Could you check a few things on this model? Use its own coordinates, in mm. A direction names the side the tool comes from. Coordinates: 2 decimals unless noted, no trailing zeros. Write each loop counter-clockwise with the first axis right and the second up, starting at its lowest first coordinate (ties: lowest second). Pieces come first, ordered by that corner, then holes. Notation, with made-up numbers: M 72.25,38 L 130.25,38 A18 cw 130.25,53 Z; hole C 3,57 d7. An arc over 180 degrees is marked long. Write item = value, one per line.
```python
from build123d import *

# Parameters (mm, degrees)
SKETCH_1_R          = 72.5
SKETCH_1_R_2        = 50
EXTRUDE_1_DEPTH     = 13
SKETCH_2_R          = 65
SKETCH_2_R_2        = 55
CUT_EXTRUDE_1_DEPTH = 10


with BuildPart() as part:
    # 草图1 → 凸台-拉伸1 (new body)
    with BuildSketch(Plane(origin=(0, 0, 0), x_dir=(1, 0, 0), z_dir=(0, 1, 0))):
        with Locations(Location((0, 0, 0), (0, 0, 90))):
            Circle(SKETCH_1_R)
        with Locations(Location((0, 0, 0), (0, 0, 90))):
            Circle(SKETCH_1_R_2, mode=Mode.SUBTRACT)
    extrude(amount=EXTRUDE_1_DEPTH)

    # 草图2 → 切除-拉伸1 (cut)
    with BuildSketch(Plane(origin=(0, 13, 0), x_dir=(1, 0, 0), z_dir=(0, 1, 0))):
        with Locations(Location((0, 0, 0), (0, 0, 270))):
            Circle(SKETCH_2_R)
        with Locations(Location((0, 0, 0), (0, 0, 270))):
            Circle(SKETCH_2_R_2, mode=Mode.SUBTRACT)
    extrude(amount=-CUT_EXTRUDE_1_DEPTH, mode=Mode.SUBTRACT)


solid = part.part
```
Item 1: For faces 4 (the face through (14.7, 3, -53.3)), 5 (the face through (-15.02, 6.41, -47.69)), which set-ups out of +Z, -Z, +X, -X, +Y, -Y let a thin tool reach every point of the face, with its end or its side?
Numbers:
face_4 = +Y
face_5 = +Y, -Y
Item 2: I'm going to push flat-ended pins straight in: P1, Ø1.5, axis at x = 6, y = 4, coming from the +Z side; P2, Ø8, axis at x = 0.5, z = 49, coming from the +Y side; P3, Ø1, axis at y = 6, z = 54.5, coming from the +X side; P4, Ø4, axis at y = 7, z = 26, coming from the +X side. Where does each tip first touch, or does it pass through?
Numbers:
P1 = 72.31
P2 = 13
P3 = 48.38
P4 = 68.41
Item 3: If we mould it in two halves opening along Z, with no side actions, what happens to faces 1 (the face through (47.3, 0, 17.1)), 2 (the face through (-48.794, 8.07, 25.379)), 3 (the face through (-21.78, 6.41, -69.15))? For each: pulls with the +Z half, pulls with the -Z half, needs draft (parallel to the pull), parting line crosses it, or undercut.
Numbers:
face_1 = needs draft
face_2 = undercut
face_3 = parting line crosses it
Item 4: Imagine slicing it at A-A (z = 0). Write out the boundary of the cut face in (x, y), and give its area (3 significant figures).
Numbers:
outline = M -72.5,0 L -50,0 L -50,13 L -55,13 L -55,3 L -65,3 L -65,13 L -72.5,13 Z; M 50,0 L 72.5,0 L 72.5,13 L 65,13 L 65,3 L 55,3 L 55,13 L 50,13 Z
area = 385 mm²
Item 5: Imagine slicing it at C-C (y = 5). Write out the boundary of the cut face in (x, z), and give its area (3 significant figures).
Numbers:
outline = C 0,0 d145; C 0,0 d110; hole C 0,0 d130; hole C 0,0 d100
area = 4,890 mm²
Item 6: Imagine slicing it at D-D (z = -57). Write out the boundary of the cut face in (x, y).
Numbers:
outline = M -44.8,0 L 44.8,0 L 44.8,13 L 31.24,13 L 31.24,3 L -31.24,3 L -31.24,13 L -44.8,13 Z
Item 7: Imagine slicing it at B-B (x = 0). Write out the boundary of the cut face in (y, z), and give its area (3 significant figures).
Numbers:
outline = M 0,-72.5 L 13,-72.5 L 13,-65 L 3,-65 L 3,-55 L 13,-55 L 13,-50 L 0,-50 Z; M 0,50 L 13,50 L 13,55 L 3,55 L 3,65 L 13,65 L 13,72.5 L 0,72.5 Z
area = 385 mm²
Item 8: If I drill on line 1 along X through (y, z) = (6, 0); line 2 along X through (y, z) = (4.5, 12); line 3 along Z through (x, y) = (18, 10), over which ranges is the centre line in solid material (lowest first)?
Numbers:
line_1 = -72.5 to -65, -55 to -50, 50 to 55, 65 to 72.5
line_2 = -71.5 to -63.88, -53.67 to -48.54, 48.54 to 53.67, 63.88 to 71.5
line_3 = -70.23 to -62.46, -51.97 to -46.65, 46.65 to 51.97, 62.46 to 70.23
